from build123d import *

# Parameters (mm, degrees)
SKETCH_1_R          = 1.6
SKETCH_1_W          = 83.5
SKETCH_1_H          = 20.5
EXTRUDE_1_DEPTH     = 2
SKETCH_3_W          = 5
SKETCH_3_H          = 10
CUT_EXTRUDE_2_DEPTH = 101.127730924
SKETCH_4_W          = 9
SKETCH_4_H          = 7
SKETCH_4_W_2        = 23
SKETCH_4_H_2        = 5.5
SKETCH_4_W_3        = 38
CUT_EXTRUDE_3_DEPTH = 101.127730924
SKETCH_5_W          = 12
SKETCH_5_H          = 4
CUT_EXTRUDE_4_DEPTH = 101.127730924
FILLET_8_R          = 2
FILLET_9_R          = 2
SKETCH_7_W          = 10
SKETCH_7_H          = 10
EXTRUDE_3_DEPTH     = 2
SKETCH_9_W          = 162.568913239
SKETCH_9_H          = 21.283892233
CUT_EXTRUDE_5_DEPTH = 103.240219581
SKETCH_8_W          = 3
SKETCH_8_H          = 6
EXTRUDE_4_DEPTH     = 2
CUT_EXTRUDE_6_DEPTH = 106.090734606
FILLET_10_R         = 5


with BuildPart() as part:
    # 草图1 → 凸台-拉伸1 (new body)
    with BuildSketch(Plane.XY):
        Polygon((64, -19.25), (29, -19.25), (29, -24.75), (-29, -24.75), (-29, -19.25), (-64, -19.25), (-64, -24.75), (-97, -24.75), (-97, 22.25), (97, 22.25), (97, -24.75), (64, -24.75), align=None)
        with Locations((-46.5, 17.25)):
            Circle(SKETCH_1_R, mode=Mode.SUBTRACT)
        with Locations((-69, -14.25)):
            Circle(SKETCH_1_R, mode=Mode.SUBTRACT)
        with Locations((-24, -14.25)):
            Circle(SKETCH_1_R, mode=Mode.SUBTRACT)
        with Locations(Location((69, -14.25, 0), (0, 0, 180))):
            Circle(SKETCH_1_R, mode=Mode.SUBTRACT)
        with Locations(Location((46.5, 17.25, 0), (0, 0, 180))):
            Circle(SKETCH_1_R, mode=Mode.SUBTRACT)
        with Locations(Location((24, -14.25, 0), (0, 0, 180))):
            Circle(SKETCH_1_R, mode=Mode.SUBTRACT)
        with Locations((-69, -21.75)):
            Circle(SKETCH_1_R, mode=Mode.SUBTRACT)
        with Locations((-24, -21.75)):
            Circle(SKETCH_1_R, mode=Mode.SUBTRACT)
        with Locations((24, -21.75)):
            Circle(SKETCH_1_R, mode=Mode.SUBTRACT)
        with Locations((69, -21.75)):
            Circle(SKETCH_1_R, mode=Mode.SUBTRACT)
        with Locations((-49.25, 0)):
            Rectangle(SKETCH_1_W, SKETCH_1_H, mode=Mode.SUBTRACT)
        with Locations((49.25, 0)):
            Rectangle(SKETCH_1_W, SKETCH_1_H, mode=Mode.SUBTRACT)
    extrude(amount=EXTRUDE_1_DEPTH)

    # 草图3 → 切除-拉伸2 (cut, through all)
    with BuildSketch(Plane.XY.offset(2)):
        with Locations((-5, 5.25)):
            Rectangle(SKETCH_3_W, SKETCH_3_H)
        with Locations((5, 5.25)):
            Rectangle(SKETCH_3_W, SKETCH_3_H)
    extrude(amount=-CUT_EXTRUDE_2_DEPTH, mode=Mode.SUBTRACT)

    # 草图4 → 切除-拉伸3 (cut, through all)
    with BuildSketch(Plane(origin=(0, 0, 0), x_dir=(-1, 0, 0), z_dir=(0, 0, -1))):
        with Locations((-69, 16.25)):
            Rectangle(SKETCH_4_W, SKETCH_4_H)
        with Locations((-24, 16.25)):
            Rectangle(SKETCH_4_W, SKETCH_4_H)
        with Locations((24, 16.25)):
            Rectangle(SKETCH_4_W, SKETCH_4_H)
        with Locations((69, 16.25)):
            Rectangle(SKETCH_4_W, SKETCH_4_H)
        with Locations((-85.5, -22)):
            Rectangle(SKETCH_4_W_2, SKETCH_4_H_2)
        with Locations((85.5, -22)):
            Rectangle(SKETCH_4_W_2, SKETCH_4_H_2)
        with Locations((0, -22)):
            Rectangle(SKETCH_4_W_3, SKETCH_4_H_2)
    extrude(amount=-CUT_EXTRUDE_3_DEPTH, mode=Mode.SUBTRACT)

    # 草图5 → 切除-拉伸4 (cut, through all)
    with BuildSketch(Plane(origin=(0, 0, 0), x_dir=(-1, 0, 0), z_dir=(0, 0, -1))):
        with Locations((-83.5, 18.25)):
            Rectangle(SKETCH_5_W, SKETCH_5_H)
        with Locations((9.5, 18.25)):
            Rectangle(SKETCH_5_W, SKETCH_5_H)
    extrude(amount=-CUT_EXTRUDE_4_DEPTH, mode=Mode.SUBTRACT)

    # 圆角8
    fillet_8_edges = [part.edges().sort_by_distance(p)[0] for p in [
        (-7.5, 0.25, 1),
        (-2.5, 10.25, 1),
        (-2.5, 0.25, 1),
        (7.5, 0.25, 1),
        (2.5, 0.25, 1),
        (2.5, 10.25, 1),
        (-91, 10.25, 1),
        (-91, -10.25, 1),
        (-7.5, -10.25, 1),
        (7.5, -10.25, 1),
        (91, -10.25, 1),
        (91, 10.25, 1),
    ]]
    fillet(fillet_8_edges, radius=FILLET_8_R)

    # 圆角9
    fillet_9_edges = [part.edges().sort_by_distance(p)[0] for p in [
        (74, -19.25, 1),
        (74, -24.75, 1),
        (-74, -24.75, 1),
        (-74, -19.25, 1),
        (19, -24.75, 1),
        (19, -19.25, 1),
        (64, -24.75, 1),
        (-19, -19.25, 1),
        (-19, -24.75, 1),
        (64, -19.25, 1),
        (29, -19.25, 1),
        (29, -24.75, 1),
        (-29, -24.75, 1),
        (-29, -19.25, 1),
        (-64, -19.25, 1),
        (-64, -24.75, 1),
    ]]
    fillet(fillet_9_edges, radius=FILLET_9_R)

    # 草图7 → 凸台-拉伸3 (add)
    with BuildSketch(Plane(origin=(0, 0, 0), x_dir=(-1, 0, 0), z_dir=(0, 0, -1))):
        with Locations((-92, 27.25)):
            Rectangle(SKETCH_7_W, SKETCH_7_H)
        with Locations((-92, -24.25)):
            Rectangle(SKETCH_7_W, SKETCH_7_H)
        with Locations((92, 27.25)):
            Rectangle(SKETCH_7_W, SKETCH_7_H)
        with Locations((92, -24.25)):
            Rectangle(SKETCH_7_W, SKETCH_7_H)
    extrude(amount=-EXTRUDE_3_DEPTH)

    # 草图9 → 切除-拉伸5 (cut, through all)
    with BuildSketch(Plane(origin=(0, 0, 0), x_dir=(-1, 0, 0), z_dir=(0, 0, -1))):
        with Locations((0.619782194, -29.891946117)):
            Rectangle(SKETCH_9_W, SKETCH_9_H)
    extrude(amount=-CUT_EXTRUDE_5_DEPTH, mode=Mode.SUBTRACT)

    # 草图8 → 凸台-拉伸4 (add)
    with BuildSketch(Plane(origin=(0, 0, 0), x_dir=(-1, 0, 0), z_dir=(0, 0, -1))):
        Polygon((-87, 32.25), (-81, 22.25), (-87, 22.25), align=None)
        Polygon((87, 32.25), (81, 22.25), (87, 22.25), align=None)
        Polygon((-87, -29.25), (-81, -19.25), (-87, -19.25), align=None)
        Polygon((87, -29.25), (81, -19.25), (87, -19.25), align=None)
        with Locations((-98.5, 16.5)):
            Rectangle(SKETCH_8_W, SKETCH_8_H)
        with Locations((-98.5, -13.5)):
            Rectangle(SKETCH_8_W, SKETCH_8_H)
        with Locations((98.5, -13.5)):
            Rectangle(SKETCH_8_W, SKETCH_8_H)
        with Locations((98.5, 16.5)):
            Rectangle(SKETCH_8_W, SKETCH_8_H)
    extrude(amount=-EXTRUDE_4_DEPTH)

    # 草图10 → 切除-拉伸6 (cut, through all)
    with BuildSketch(Plane(origin=(0, 0, 0), x_dir=(-1, 0, 0), z_dir=(0, 0, -1))):
        Polygon((-97, 27.85), (-93, 27.85), (-93, 29.25), (-90, 29.25), (-90, 27.85), (-88, 27.85), (-88, 24.65), (-90, 24.65), (-90, 23.25), (-93, 23.25), (-93, 24.65), (-97, 24.65), align=None)
        Polygon((-97, -24.85), (-93, -24.85), (-93, -26.25), (-90, -26.25), (-90, -24.85), (-88, -24.85), (-88, -21.65), (-90, -21.65), (-90, -20.25), (-93, -20.25), (-93, -21.65), (-97, -21.65), align=None)
        Polygon((97, -24.85), (97, -21.65), (93, -21.65), (93, -20.25), (90, -20.25), (90, -21.65), (88, -21.65), (88, -24.85), (90, -24.85), (90, -26.25), (93, -26.25), (93, -24.85), align=None)
        Polygon((97, 27.85), (93, 27.85), (93, 29.25), (90, 29.25), (90, 27.85), (88, 27.85), (88, 24.65), (90, 24.65), (90, 23.25), (93, 23.25), (93, 24.65), (97, 24.65), align=None)
    extrude(amount=-CUT_EXTRUDE_6_DEPTH, mode=Mode.SUBTRACT)

    # 圆角10
    fillet_10_edges = [part.edges().sort_by_distance(p)[0] for p in [
        (87, 32.25, 1),
        (87, -29.25, 1),
        (-87, 32.25, 1),
        (-87, -29.25, 1),
        (81, 22.25, 1),
        (-81, 22.25, 1),
        (81, -19.25, 1),
        (-81, -19.25, 1),
    ]]
    fillet(fillet_10_edges, radius=FILLET_10_R)


solid = part.part
Check sheet for the modelled part. Datum: model origin and axes. Units: mm. Round coordinates to 2 decimals unless told otherwise and drop trailing zeros. Write each loop counter-clockwise with the first axis right and the second up, starting at its lowest first coordinate (ties: lowest second). Pieces come first, ordered by that corner, then holes. Notation, with made-up numbers: (11, 55.25) - (31, 55.25) arc R22 ccw to (31, 63.25) - close; hole circle Ø4 at (-4.75, 76.5). An arc over 180 degrees is marked (long way). Return JSON: item names as keys, results as strings.
Q1. Scan lines: L1, parallel to Y at x = -24, z = 0.45; L2, parallel to X at y = 6, z = 0.1; L3, parallel to X at y = -2.5, z = 1.25. Record each from-to range of solid material in increasing order. Write a range as from..to.
Returned:
{"L1": "y = -19.25..-15.85, -12.65..-10.25, 10.25..12.75, 19.75..22.25", "L2": "x = -97..-91, -2.5..2.5, 91..97", "L3": "x = -97..-91, -7.5..7.5, 91..97"}
Q2. Draft check along Y on faces 1 (the cylindrical face through (-45.64, 18.6, 0.99)), 2 (the flat face through (-1, -5, 0)). Enter one of: released by +Y, released by -Y, zero draft, split by the parting line, or undercut.
Returned:
{"face 1": "undercut", "face 2": "zero draft"}
Q3. Cross-section at B-B (z = 0.9). Give the number of separate pieces and of enclosed holes in the cut face, then the cut area to 3 significant figures.
Returned:
{"separate pieces": "1", "enclosed holes": "14", "area": "4,580 mm²"}
Q4. Depth check by flat-ended pin: P1, Ø0.6, axis at x = -12, z = 1.5, coming from the +Y side; P2, Ø2.5, axis at x = -24, y = -14.25, coming from the -Z side; P3, Ø1, axis at y = -26.5, z = 1.5, coming from the -X side; P4, Ø0.6, axis at x = 88.5, z = 1, coming from the +Y side. Enter the tip coordinate at first touch or a pass-through.
Returned:
{"P1": "stops at y = 22.25", "P2": "passes through", "P3": "stops at x = -97", "P4": "stops at y = 32.14"}
Q5. Cross-section at A-A (y = -4.5). Record the boundary of the cut face in (x, z), then the cut area to 3 significant figures.
Returned:
{"outline": "(-97, 0) - (-91, 0) - (-91, 2) - (-97, 2) - close; (-7.5, 0) - (7.5, 0) - (7.5, 2) - (-7.5, 2) - close; (91, 0) - (97, 0) - (97, 2) - (91, 2) - close", "area": "54.0 mm²"}
